Can you work these out from the model? Positions are in its coordinate system, mm. Face numbers are marked on the shaded views. A direction names the side the tool comes from. Coordinates: 2 decimals unless noted, no trailing zeros. Order: outer loops, then holes, each group sorted by start corner. A loop starts at its lowest first (then second) coordinate and runs counter-clockwise, first axis right, second up. Notation, with made-up numbers: (28.5, 82) -> (38.5, 82) arc R20 cw to (38.5, 118) -> close; hole circle Ø2 at (-38.5, -12). An arc over 180 degrees is marked (long way). Answer as a JSON object with one key per item and string values. Group by question number.
(1) I want a section at A-A, the plane x = 37.5. List the corners of the cut face in (y, z) for me.
(2) For pin 1 (0.8 mm diameter, centred on x = -29.5, z = -16, fed in from +Y); pin 2 (5 mm diameter, centred on x = -29, z = -3, fed in from +Y); pin 3 (4.5 mm diameter, centred on y = 5.5, z = 4.5, fed in from +X), each with a flat end and sliding along its axis, tell me the tip position at first contact or that it passes through.
(3) I want a section at B-B, the plane z = -6. List the corners of the cut face in (x, y) for me.
(4) Which directions (+Z, -Z, +X, -X, +Y, -Y) give clear straight access to the entire face, cutting with the end or side of a thin tool? Please do the marked faces 5 and 6.
(5) I want a section at C-C, the plane y = -7.5. List the corners of the cut face in (x, z) for me.
(6) I want a section at D-D, the plane x = 11. List the corners of the cut face in (y, z) for me.
(7) If we mould it in two halves opening along Z, with no side actions, what happens to the marked faces 1, 2, 3 and 4? For each: pulls with the +Z half, pulls with the -Z half, needs draft (parallel to the pull), parting line crosses it, or undercut.
(8) I need wall thicknesses on line 1 (Z direction, x = -37.5, y = 0.45); line 2 (X direction, y = 1.05, z = 15.5); line 3 (Y direction, x = 5, z = -6.5). Which ranges of each line are inside material? Lowest first, please.
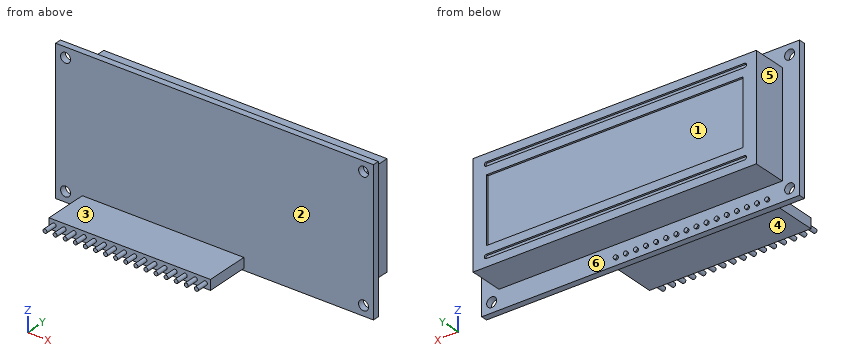
from build123d import *

# Parameters (mm, degrees)
SKETCH1_W                = 80
SKETCH1_H                = 36
SKETCH1_R                = 1.25
SKETCH1_R_2              = 0.5
BOSS_EXTRUDE1_DEPTH      = 1.6
SKETCH2_W                = 71.3
SKETCH2_H                = 26.3
BOSS_EXTRUDE2_DEPTH      = 8.6
SKETCH3_W                = 64.5
SKETCH3_H                = 16.4
CUT_EXTRUDE1_DEPTH       = 0.5
CUT_EXTRUDE2_DEPTH       = 0.5
SKETCH5_W                = 40.64
SKETCH5_H                = 2.54
BOSS_EXTRUDE3_DEPTH      = 2.54
SKETCH6_R                = 0.5
BOSS_EXTRUDE4_DEPTH      = 11.5
BOSS_EXTRUDE4_DEPTH_BACK = 4.54
SKETCH7_W                = 40.64
SKETCH7_H                = 2.54
BOSS_EXTRUDE5_DEPTH      = 8.5


with BuildPart() as part:
    # Sketch1 → Boss-Extrude1 (new body)
    with BuildSketch(Plane(origin=(0, 0, 0), x_dir=(1, 0, 0), z_dir=(0, 1, 0))):
        Rectangle(SKETCH1_W, SKETCH1_H)
        with Locations((-37.5, 15.5)):
            Circle(SKETCH1_R, mode=Mode.SUBTRACT)
        with Locations((37.5, 15.5)):
            Circle(SKETCH1_R, mode=Mode.SUBTRACT)
        with Locations((37.5, -15.5)):
            Circle(SKETCH1_R, mode=Mode.SUBTRACT)
        with Locations((-37.5, -15.5)):
            Circle(SKETCH1_R, mode=Mode.SUBTRACT)
        with Locations((-32, 16.25)):
            Circle(SKETCH1_R_2, mode=Mode.SUBTRACT)
        with Locations((-29.46, 16.25)):
            Circle(SKETCH1_R_2, mode=Mode.SUBTRACT)
        with Locations((-26.92, 16.25)):
            Circle(SKETCH1_R_2, mode=Mode.SUBTRACT)
        with Locations((-24.38, 16.25)):
            Circle(SKETCH1_R_2, mode=Mode.SUBTRACT)
        with Locations((-21.84, 16.25)):
            Circle(SKETCH1_R_2, mode=Mode.SUBTRACT)
        with Locations((-19.3, 16.25)):
            Circle(SKETCH1_R_2, mode=Mode.SUBTRACT)
        with Locations((-16.76, 16.25)):
            Circle(SKETCH1_R_2, mode=Mode.SUBTRACT)
        with Locations((-14.22, 16.25)):
            Circle(SKETCH1_R_2, mode=Mode.SUBTRACT)
        with Locations((-11.68, 16.25)):
            Circle(SKETCH1_R_2, mode=Mode.SUBTRACT)
        with Locations((-9.14, 16.25)):
            Circle(SKETCH1_R_2, mode=Mode.SUBTRACT)
        with Locations((-6.6, 16.25)):
            Circle(SKETCH1_R_2, mode=Mode.SUBTRACT)
        with Locations((-4.06, 16.25)):
            Circle(SKETCH1_R_2, mode=Mode.SUBTRACT)
        with Locations((-1.52, 16.25)):
            Circle(SKETCH1_R_2, mode=Mode.SUBTRACT)
        with Locations((1.02, 16.25)):
            Circle(SKETCH1_R_2, mode=Mode.SUBTRACT)
        with Locations((3.56, 16.25)):
            Circle(SKETCH1_R_2, mode=Mode.SUBTRACT)
        with Locations((6.1, 16.25)):
            Circle(SKETCH1_R_2, mode=Mode.SUBTRACT)
    extrude(amount=BOSS_EXTRUDE1_DEPTH)

    # Sketch2 → Boss-Extrude2 (add)
    with BuildSketch(Plane(origin=(0, 1.6, 0), x_dir=(1, 0, 0), z_dir=(0, 1, 0))):
        Rectangle(SKETCH2_W, SKETCH2_H)
    extrude(amount=BOSS_EXTRUDE2_DEPTH)

    # Sketch3 → Cut-Extrude1 (cut)
    with BuildSketch(Plane(origin=(0, 10.2, 0), x_dir=(1, 0, 0), z_dir=(0, 1, 0))):
        Rectangle(SKETCH3_W, SKETCH3_H)
    extrude(amount=-CUT_EXTRUDE1_DEPTH, mode=Mode.SUBTRACT)

    # Sketch4 → Cut-Extrude2 (cut)
    with BuildSketch(Plane(origin=(0, 10.2, 0), x_dir=(1, 0, 0), z_dir=(0, 1, 0))):
        with BuildLine():
            Line((-32.681461103, 10.2), (32.318538897, 10.2))
            ThreePointArc((32.318538897, 10.2), (32.818538897, 10.7), (32.318538897, 11.2))
            Line((32.318538897, 11.2), (-32.681461103, 11.2))
            ThreePointArc((-32.681461103, 11.2), (-33.181461103, 10.7), (-32.681461103, 10.2))
        make_face()
    cut_extrude2 = extrude(amount=-CUT_EXTRUDE2_DEPTH, mode=Mode.SUBTRACT)

    # Mirror1: Cut-Extrude2 across plane
    add(cut_extrude2.mirror(Plane.XY), mode=Mode.SUBTRACT)

    # Sketch5 → Boss-Extrude3 (add)
    with BuildSketch(Plane.XZ):
        with Locations((-12.95, -16.25)):
            Rectangle(SKETCH5_W, SKETCH5_H)
    extrude(amount=BOSS_EXTRUDE3_DEPTH)

    # Sketch6 → Boss-Extrude4 (add, two sides)
    with BuildSketch(Plane.XZ.offset(2.54)) as boss_extrude4_sk:
        with Locations((-32, -16.25)):
            Circle(SKETCH6_R)
        with Locations((-29.46, -16.25)):
            Circle(SKETCH6_R)
        with Locations((-26.92, -16.25)):
            Circle(SKETCH6_R)
        with Locations((-24.38, -16.25)):
            Circle(SKETCH6_R)
        with Locations((-21.84, -16.25)):
            Circle(SKETCH6_R)
        with Locations((-19.3, -16.25)):
            Circle(SKETCH6_R)
        with Locations((-16.76, -16.25)):
            Circle(SKETCH6_R)
        with Locations((-14.22, -16.25)):
            Circle(SKETCH6_R)
        with Locations((-11.68, -16.25)):
            Circle(SKETCH6_R)
        with Locations((-9.14, -16.25)):
            Circle(SKETCH6_R)
        with Locations((-6.6, -16.25)):
            Circle(SKETCH6_R)
        with Locations((-4.06, -16.25)):
            Circle(SKETCH6_R)
        with Locations((-1.52, -16.25)):
            Circle(SKETCH6_R)
        with Locations((1.02, -16.25)):
            Circle(SKETCH6_R)
        with Locations((3.56, -16.25)):
            Circle(SKETCH6_R)
        with Locations((6.1, -16.25)):
            Circle(SKETCH6_R)
    extrude(amount=BOSS_EXTRUDE4_DEPTH)
    extrude(boss_extrude4_sk.sketch, amount=-BOSS_EXTRUDE4_DEPTH_BACK)

    # Sketch7 → Boss-Extrude5 (add)
    with BuildSketch(Plane.XZ.offset(2.54)):
        with Locations((-12.95, -16.25)):
            Rectangle(SKETCH7_W, SKETCH7_H)
    extrude(amount=BOSS_EXTRUDE5_DEPTH)


solid = part.part
Computed values:
{
 "1": {"outline": "(0, -18) -> (1.6, -18) -> (1.6, -16.75) -> (0, -16.75) -> close; (0, -14.25) -> (1.6, -14.25) -> (1.6, 14.25) -> (0, 14.25) -> close; (0, 16.75) -> (1.6, 16.75) -> (1.6, 18) -> (0, 18) -> close"},
 "2": {"pin 1": "stops at y = 2", "pin 2": "stops at y = 9.7", "pin 3": "stops at x = 35.65"},
 "3": {"outline": "(-40, 0) -> (40, 0) -> (40, 1.6) -> (35.65, 1.6) -> (35.65, 10.2) -> (32.25, 10.2) -> (32.25, 9.7) -> (-32.25, 9.7) -> (-32.25, 10.2) -> (-35.65, 10.2) -> (-35.65, 1.6) -> (-40, 1.6) -> close"},
 "4": {"face 5": "+Z, -Z, -X, +Y", "face 6": "+Y"},
 "5": {"outline": "(-33.27, -17.52) -> (7.37, -17.52) -> (7.37, -14.98) -> (-33.27, -14.98) -> close"},
 "6": {"outline": "(0, -18) -> (1.6, -18) -> (1.6, -13.15) -> (10.2, -13.15) -> (10.2, -11.2) -> (9.7, -11.2) -> (9.7, -10.2) -> (10.2, -10.2) -> (10.2, -8.2) -> (9.7, -8.2) -> (9.7, 8.2) -> (10.2, 8.2) -> (10.2, 10.2) -> (9.7, 10.2) -> (9.7, 11.2) -> (10.2, 11.2) -> (10.2, 13.15) -> (1.6, 13.15) -> (1.6, 18) -> (0, 18) -> close"},
 "7": {"face 1": "undercut", "face 2": "needs draft", "face 3": "pulls with the +Z half", "face 4": "pulls with the -Z half"},
 "8": {"line 1": "z = -18 to -16.75, -14.25 to 14.25, 16.75 to 18", "line 2": "x = -40 to -38.75, -36.25 to 36.25, 38.75 to 40", "line 3": "y = 0 to 9.7"}
}
